The drawing under review shows one solid part. Ordinate dimensions are in mm from its lowest x, y, z. Give positions to 0.01 mm unless a question says otherwise; leave off trailing zeros. Loops run counter-clockwise (first coordinate to the right, second up) from the corner with the lowest first, then second, coordinate; pieces in that order, holes last. Notation, with made-up numbers: (54.25, -2) -> (72.25, -2) arc R33 ccw to (72.25, 36) -> close; hole circle Ø1 at (-1.5, 62.5). An arc over 180 degrees is marked (long way). Answer in a Markdown table with one row per item. Add a question column.
(1) Consider section C-C on y = 5.25. Write out the cut boundary in (x, z).
(2) For pin 1 (1 mm diameter, centred on x = 17, y = 5, fed in from -Z); pin 2 (1.5 mm diameter, centred on x = 20.5, y = 1.5, fed in from +Z); pin 3 (8 mm diameter, centred on x = 22.5, z = 9.5, fed in from -Y); pin 4 (4 mm diameter, centred on x = 15, z = 14, fed in from +Y), all flat-tipped, find the tip position at first contact; note any pin that passes through.
(3) Consider section A-A on z = 14. Write out the cut boundary in (x, y), then the cut area to 3 significant figures.
(4) Draft analysis for pull direction X (two halves, no side actions). For the marked faces 1, 2 and 3, state which applies: +X half, -X half, draft (parallel to the pull), parting line (faces both ways), or undercut.
(5) Consider section B-B on x = 16. Write out the cut boundary in (y, z).
(6) For line 1 (Z direction, x = 15, y = 4.5); line 2 (Z direction, x = 14.5, y = 5); line 3 (X direction, y = 4.5, z = 14), list the stretches that pass through material, from the lowest coordinate up.
(7) Consider section D-D on z = 4.75. Write out the cut boundary in (x, y).
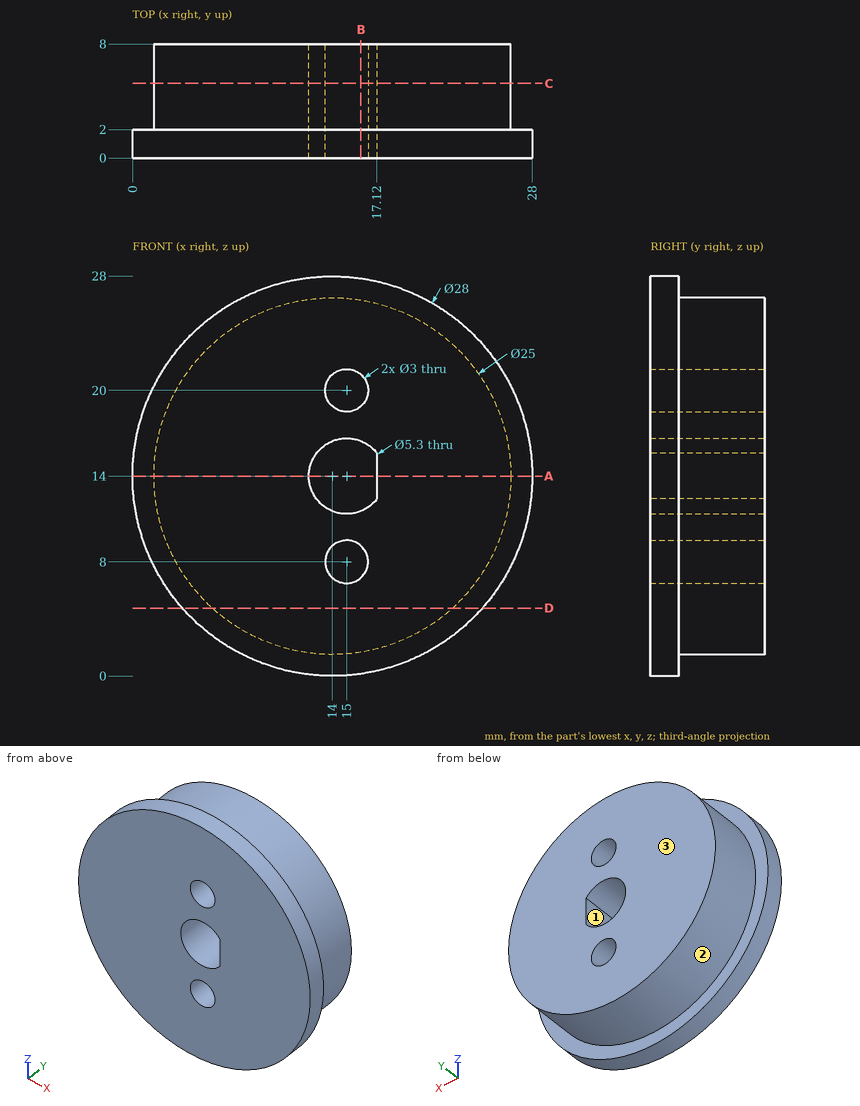
Values follow:
| question | item | result |
|---|---|---|
| 1 | outline | circle Ø25 at (14, 14); hole circle Ø3 at (15, 8); hole circle Ø3 at (15, 20); hole (17.12, 12.41) -> (17.12, 15.59) arc R2.65 ccw (long way) to start |
| 2 | pin 1 | z = 1.75 |
| 2 | pin 2 | z = 26.76 |
| 2 | pin 3 | y = 0 |
| 2 | pin 4 | through |
| 3 | outline | (0, 0) -> (12.35, 0) -> (12.35, 8) -> (1.5, 8) -> (1.5, 2) -> (0, 2) -> close; (17.12, 0) -> (28, 0) -> (28, 2) -> (26.5, 2) -> (26.5, 8) -> (17.12, 8) -> close |
| 3 | area | 168 mm2 |
| 4 | face 1 | undercut |
| 4 | face 2 | parting line |
| 4 | face 3 | draft |
| 5 | outline | (0, 0.14) -> (2, 0.14) -> (2, 1.66) -> (8, 1.66) -> (8, 6.88) -> (0, 6.88) -> close; (0, 9.12) -> (8, 9.12) -> (8, 11.55) -> (0, 11.55) -> close; (0, 16.45) -> (8, 16.45) -> (8, 18.88) -> (0, 18.88) -> close; (0, 21.12) -> (8, 21.12) -> (8, 26.34) -> (2, 26.34) -> (2, 27.86) -> (0, 27.86) -> close |
| 6 | line 1 | 1.54 to 6.5, 9.5 to 11.35, 16.65 to 18.5, 21.5 to 26.46 |
| 6 | line 2 | 1.51 to 6.59, 9.41 to 11.4, 16.6 to 18.59, 21.41 to 26.49 |
| 6 | line 3 | 1.5 to 12.35, 17.12 to 26.5 |
| 7 | outline | (3.49, 0) -> (24.51, 0) -> (24.51, 2) -> (22.41, 2) -> (22.41, 8) -> (5.59, 8) -> (5.59, 2) -> (3.49, 2) -> close |
